CAD build for the part. Positions are in the model's coordinates, mm. A direction names the side the tool comes from. Give positions to 0.01 mm unless a question says otherwise; leave off trailing zeros. Loops run counter-clockwise (first coordinate to the right, second up) from the corner with the lowest first, then second, coordinate; pieces in that order, holes last.
```python
from build123d import *

# Parameters (mm, degrees)
SKETCH2_R           = 5
BOSS_EXTRUDE1_DEPTH = 44
SKETCH4_R           = 7
CUT_EXTRUDE1_DEPTH  = 44
SKETCH3_R           = 15
SKETCH3_R_2         = 1.432268471
SKETCH3_R_3         = 1.5
CUT_EXTRUDE2_DEPTH  = 8.5


with BuildPart() as part:
    # Sketch2 → Boss-Extrude1 (new body)
    with BuildSketch(Plane(origin=(0, 5.184806561, 52.754021043), x_dir=(1, 0, 0), z_dir=(0, 0.097811411, 0.995204968))):
        with BuildLine():
            Line((-79.338568196, 60.019636282), (-86.171283653, 157.182642502))
            ThreePointArc((-86.171283653, 157.182642502), (-85.540604549, 159.070011115), (-83.760075933, 159.958624788))
            Line((-83.760075933, 159.958624788), (-66.40294057, 161.179216572))
            ThreePointArc((-66.40294057, 161.179216572), (-63.499296447, 160.208940992), (-62.13219844, 157.469666101))
            Line((-62.13219844, 157.469666101), (-59.185942386, 115.573132123))
            Line((-59.185942386, 115.573132123), (-58.165469, 72.72467593))
            ThreePointArc((-58.165469, 72.72467593), (-56.858994047, 69.861695577), (-53.88600747, 68.829763352))
            Line((-53.88600747, 68.829763352), (-37.927916785, 69.95197125))
            ThreePointArc((-37.927916785, 69.95197125), (-34.211684563, 68.662057426), (-32.578589401, 65.083334219))
            Line((-32.578589401, 65.083334219), (-31.866862588, 35.198777134))
            ThreePointArc((-31.866862588, 35.198777134), (-32.387188107, 33.80496391), (-33.725997726, 33.156085835))
            Line((-33.725997726, 33.156085835), (-57.666874392, 31.472510939))
            ThreePointArc((-57.666874392, 31.472510939), (-59.969896102, 31.85708433), (-61.84718043, 33.245468007))
            Line((-61.84718043, 33.245468007), (-74.706082713, 48.563713079))
            ThreePointArc((-74.706082713, 48.563713079), (-77.929269747, 53.924929356), (-79.338568196, 60.019636282))
        make_face()
        with Locations((-43.960887699, 60.004258737)):
            Circle(SKETCH2_R, mode=Mode.SUBTRACT)
        with BuildLine():
            Line((-62.966135351, 68.191231545), (-74.842135577, 67.356085192))
            ThreePointArc((-74.842135577, 67.356085192), (-76.293957569, 67.841222959), (-76.97750654, 69.21086034))
            Line((-76.97750654, 69.21086034), (-77.398400264, 75.196079506))
            ThreePointArc((-77.398400264, 75.196079506), (-76.913262497, 76.647901499), (-75.543625116, 77.33145047))
            Line((-75.543625116, 77.33145047), (-63.389739784, 78.186138312))
            ThreePointArc((-63.389739784, 78.186138312), (-61.903246895, 77.670172783), (-61.25000883, 76.2386835))
            Line((-61.25000883, 76.2386835), (-61.107000214, 70.233922844))
            ThreePointArc((-61.107000214, 70.233922844), (-61.627325733, 68.84010962), (-62.966135351, 68.191231545))
        make_face(mode=Mode.SUBTRACT)
        with BuildLine():
            Line((-63.800352281, 103.21900204), (-77.297348966, 102.269863664))
            ThreePointArc((-77.297348966, 102.269863664), (-78.749170958, 102.755001431), (-79.43271993, 104.124638812))
            Line((-79.43271993, 104.124638812), (-79.993911561, 112.104931034))
            ThreePointArc((-79.993911561, 112.104931034), (-79.508773795, 113.556753027), (-78.139136414, 114.240301998))
            Line((-78.139136414, 114.240301998), (-64.271626252, 115.215495692))
            ThreePointArc((-64.271626252, 115.215495692), (-62.785133364, 114.699530163), (-62.131895299, 113.26804088))
            Line((-62.131895299, 113.26804088), (-61.941217144, 105.261693339))
            ThreePointArc((-61.941217144, 105.261693339), (-62.461542663, 103.867880114), (-63.800352281, 103.21900204))
        make_face(mode=Mode.SUBTRACT)
        with BuildLine():
            Line((-76.689803818, 136.396552471), (-77.391293358, 146.371917749))
            ThreePointArc((-77.391293358, 146.371917749), (-77.167089785, 147.441743104), (-76.413930361, 148.233920114))
            Line((-76.413930361, 148.233920114), (-72.564082157, 150.509588985))
            ThreePointArc((-72.564082157, 150.509588985), (-70.616844652, 150.558754011), (-69.551299044, 148.928182436))
            Line((-69.551299044, 148.928182436), (-68.709511596, 136.957744103))
            Line((-68.709511596, 136.957744103), (-67.867724148, 124.987305769))
            ThreePointArc((-67.867724148, 124.987305769), (-68.694580699, 123.223656329), (-70.629534734, 122.999817141))
            Line((-70.629534734, 122.999817141), (-74.759978753, 124.71429438))
            ThreePointArc((-74.759978753, 124.71429438), (-75.616592755, 125.393268596), (-75.988314278, 126.421187193))
            Line((-75.988314278, 126.421187193), (-76.689803818, 136.396552471))
        make_face(mode=Mode.SUBTRACT)
        with BuildLine():
            Line((-63.41899597, 87.206306956), (-76.174965702, 86.30927922))
            ThreePointArc((-76.174965702, 86.30927922), (-77.626787695, 86.794416987), (-78.310336666, 88.164054367))
            Line((-78.310336666, 88.164054367), (-78.871528298, 96.14434659))
            ThreePointArc((-78.871528298, 96.14434659), (-78.386390531, 97.596168582), (-77.01675315, 98.279717553))
            Line((-77.01675315, 98.279717553), (-63.890269942, 99.202800609))
            ThreePointArc((-63.890269942, 99.202800609), (-62.403777053, 98.68683508), (-61.750538988, 97.255345797))
            Line((-61.750538988, 97.255345797), (-61.559860833, 89.248998255))
            ThreePointArc((-61.559860833, 89.248998255), (-62.080186352, 87.855185031), (-63.41899597, 87.206306956))
        make_face(mode=Mode.SUBTRACT)
    extrude(amount=BOSS_EXTRUDE1_DEPTH)

    # Sketch4 → Cut-Extrude1 (cut)
    with BuildSketch(Plane(origin=(-74.74821025, -5.231253014, 0.514141565), x_dir=(0.006844627, 0.000479021, 0.999976461), z_dir=(-0.997536528, -0.069812587, 0.006861368))):
        with Locations((60.947145558, 147.088883585)):
            Circle(SKETCH4_R)
    extrude(amount=-CUT_EXTRUDE1_DEPTH, mode=Mode.SUBTRACT)

    # Sketch3 → Cut-Extrude2 (cut)
    with BuildSketch(Plane(origin=(-50.807333583, -3.555750914, 0.349468729), x_dir=(-0.006844627, -0.000479021, -0.999976461), z_dir=(0.997536528, 0.069812587, -0.006861368))):
        with Locations((-60.947145558, 147.088883585)):
            Circle(SKETCH3_R)
        with Locations((-74.548623077, 131.340873995)):
            Circle(SKETCH3_R_2)
        with Locations((-78.140713739, 94.702052828)):
            Circle(SKETCH3_R_3)
        with Locations((-54.255232262, 92.360306772)):
            Circle(SKETCH3_R_3)
        with Locations((-50.6631416, 128.999127938)):
            Circle(SKETCH3_R_2)
    extrude(amount=-CUT_EXTRUDE2_DEPTH, mode=Mode.SUBTRACT)


solid = part.part
```
1. Saw through at A-A, the plane z = 61. Count the separate pieces of the cut face and the enclosed holes in it, and give its area (3 significant figures).
Responses:
separate pieces: 2
enclosed holes: 4
area: 2,490 mm2
2. Pull direction X, two halves, no side cores. Call faces 5 (the face through (-68.19, 47.91, 70.35)), 6 (the face through (-46.019, 76.357, 67.556)), 7 (the face through (-45.529, 39.478, 71.18)), 8 (the face through (-64.121, 133.812, 73.227)): released by +X, released by -X, zero draft, split by the parting line, or undercut.
Responses:
face 5: released by -X
face 6: undercut
face 7: released by +X
face 8: undercut
3. Saw through at B-B, the plane x = -52.5. List the corners of the cut face in (y, z), and give its area (3 significant figures).
Responses:
outline: (36.87, 49.64) - (73.78, 46.01) - (78.09, 89.8) - (41.17, 93.43) - close
area: 1,630 mm2
4. Probe line 1 along Y through (x, z) = (-74, 74); line 2 along Y through (x, z) = (-65, 79.5); line 3 along X through (y, z) = (79, 65). List the from-to ranges inside material, lowest first.
Responses:
line 1: y = 55.23 to 75.01, 85.09 to 94.15, 106.24 to 110.27, 122.36 to 132.27, 157.65 to 168.69
line 2: y = 44.99 to 76.19, 86.26 to 89.23, 91.54 to 95.33, 107.42 to 111.45, 123.53 to 169.62
line 3: x = -80.2 to -77.19, -61.16 to -58.13
5. Drop flat-ended pins along their axis: pin 1 (4 mm diameter, centred on x = -38, z = 58, fed in from -Y); pin 2 (3 mm diameter, centred on x = -54, z = 59, fed in from -Y); pin 3 (8 mm diameter, centred on y = 148.5, z = 73, fed in from +X). Give the stop position or say it passes through.
Responses:
pin 1: stops at y = 38.47
pin 2: stops at y = 37.5
pin 3: stops at x = -60.75
6. Tool access for faces 1 (the face through (-78.4, 104.42, 64.8)), 2 (the face through (-56.89, 76.86, 67.51)), 3 (the face through (-70.642, 157.156, 59.614)), 4 (the face through (-58.642, 87.606, 44.653)): list every direction of +Z, -Z, +X, -X, +Y, -Y with a clear straight run to the whole face (end or side of a thin tool).
Responses:
face 1: none
face 2: -Z, +Y
face 3: +Z
face 4: -Z, +X, -X, -Y
7. Saw through at C-C, the plane y = 50.5. List the corners of the cut face in (x, z).
Responses:
outline: (-72.16, 48.3) - (-32.11, 48.3) - (-32.01, 92.51) - (-68.53, 92.51) - close
